The drawing under review shows one solid part. Ordinate dimensions are in mm from its lowest x, y, z. A direction names the side the tool comes from. Give positions to 0.01 mm unless a question says otherwise; leave off trailing zeros. Loops run counter-clockwise (first coordinate to the right, second up) from the corner with the lowest first, then second, coordinate; pieces in that order, holes last.
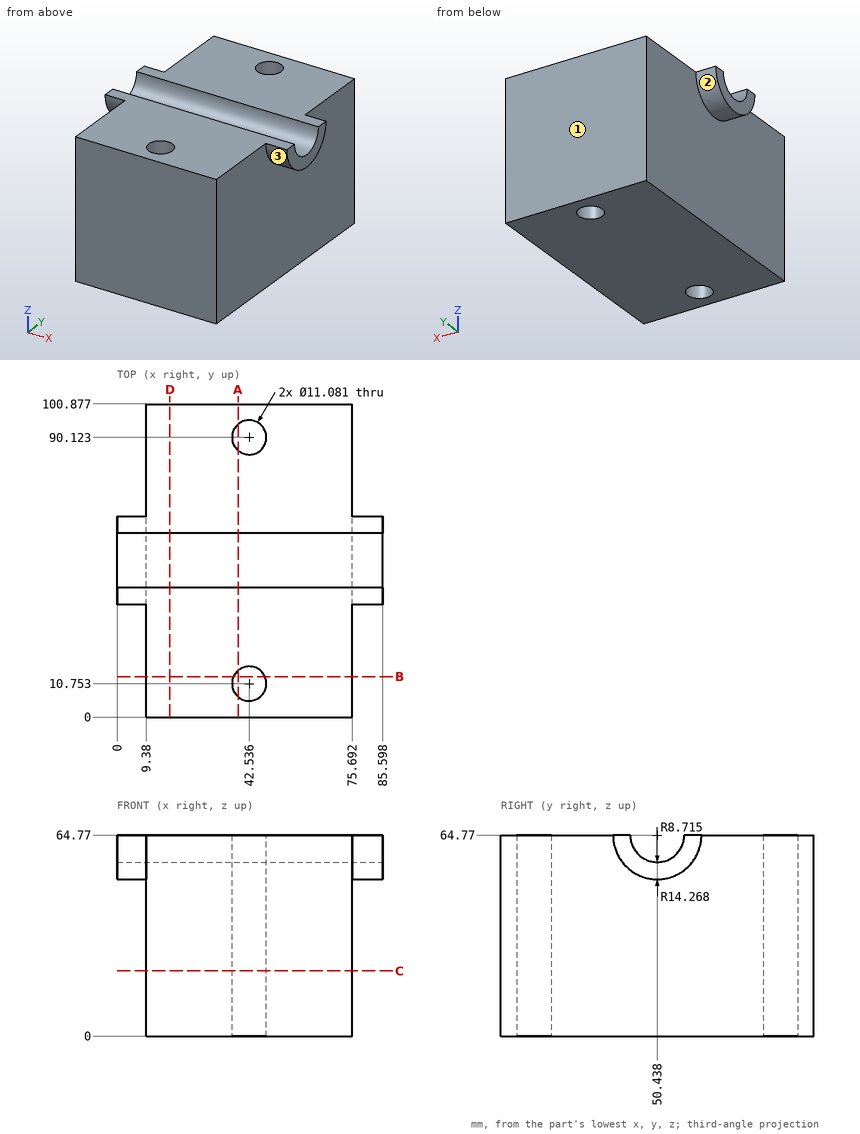
Item 1: Take a section at A-A on x = 39. Give the boundary of the cut face in (y, z) (1 decimal).
Answer:
outline: (0, 0) - (6.5, 0) - (6.5, 64.8) - (0, 64.8) - close; (15, 0) - (85.9, 0) - (85.9, 64.8) - (59.2, 64.8) arc R8.7 cw to (41.7, 64.8) - (15, 64.8) - close; (94.4, 0) - (100.9, 0) - (100.9, 64.8) - (94.4, 64.8) - close
Item 2: Take a section at B-B on y = 13. Give the boundary of the cut face in (x, z).
Answer:
outline: (9.38, 0) - (37.47, 0) - (37.47, 64.77) - (9.38, 64.77) - close; (47.6, 0) - (75.69, 0) - (75.69, 64.77) - (47.6, 64.77) - close
Item 3: Clearance check with a flat-ended pin moving along its axis: pin 1 Ø19.5 at (y, z) = (53, 18.5) entering from +X. State where the tip first meets the part, or that it passes through.
Answer:
pin 1: stops at x = 75.69
Item 4: Take a section at C-C on z = 21. Give the boundary of the cut face in (x, y), and give its area (3 significant figures).
Answer:
outline: (9.38, 0) - (75.69, 0) - (75.69, 100.88) - (9.38, 100.88) - close; hole circle Ø11.08 at (42.54, 10.75); hole circle Ø11.08 at (42.54, 90.12)
area: 6,500 mm2
Item 5: Take a section at D-D on x = 17. Give the boundary of the cut face in (y, z) (1 decimal), and give its area (3 significant figures).
Answer:
outline: (0, 0) - (100.9, 0) - (100.9, 64.8) - (59.2, 64.8) arc R8.7 cw to (41.7, 64.8) - (0, 64.8) - close
area: 6,410 mm2
Item 6: For L1, parallel to Y at x = 43.5, z = 18; L2, parallel to X at y = 25, z = 26; L3, parallel to X at y = 86.5, z = 54 (1 decimal), list the stretches that pass through material, from the lowest coordinate up.
Answer:
L1: y = 0 to 5.3, 16.21 to 84.67, 95.58 to 100.88
L2: x = 9.38 to 75.69
L3: x = 9.4 to 38.3, 46.7 to 75.7
Item 7: Tool access review of the marked faces 1, 2 and 3: name each direction out of +Z, -Z, +X, -X, +Y, -Y from which nothing blocks a thin tool from reaching the whole face with its end or side.
Answer:
face 1: +Z, -Z, +X, -X, +Y
face 2: -Z, -X
face 3: -Z, +X
